Check sheet for the modelled part. Datum: model origin and axes. Units: mm. A direction names the side the tool comes from. Coordinates: 2 decimals unless noted, no trailing zeros. Write each loop counter-clockwise with the first axis right and the second up, starting at its lowest first coordinate (ties: lowest second). Pieces come first, ordered by that corner, then holes. Notation, with made-up numbers: (-32, 19.5) - (-22, 19.5) arc R15 ccw to (-22, 48.5) - close; hole circle Ø10 at (-28, 9.25). An arc over 180 degrees is marked (long way). Use one line per item in the form item = value. Start each with the question number.
1. Scan lines: line 1 along Y through (x, z) = (35.3, -15); line 2 along Y through (x, z) = (13, -10.5); line 3 along X through (y, z) = (7, -27). Record each from-to range of solid material in increasing order.
2. Cross-section at D-D on z = -19.75. Record the boundary of the cut face in (x, y), then the cut area to 3 significant figures.
3. Tool access check on faces 1 (the face through (22, 3, -15)), 2 (the face through (33.8, -12, -15)), 3 (the face through (3, 30.65, -15)). Record the directions out of +Z, -Z, +X, -X, +Y, -Y that give a thin tool (end or side, any length) a straight path to the whole face; none if there is none.
4. Draft check along Z on faces 4 (the face through (38.048, 2.287, -15.21)), 5 (the face through (15, 2, -30)), 6 (the face through (36.265, -5.159, -18.233)), 7 (the face through (2.47, 20.99, -13.26)). Enter one of: +Z half, -Z half, draft (parallel to the pull), parting line (faces both ways), or undercut.
5. Cross-section at A-A on y = 19.65. Record the boundary of the cut face in (x, z), then the cut area to 3 significant figures.
6. Go/stop test with flat-tipped pins: pin 1 Ø12.5 at (y, z) = (17, -18) entering from +X; pin 2 Ø14.5 at (x, z) = (19.5, -13.5) entering from +Y; pin 3 Ø1 at (x, z) = (14.5, -13.5) entering from -Y. Record where each tip stops, or that it passes through.
7. Cross-section at B-B on z = -15. Record the boundary of the cut face in (x, y), then the cut area to 3 significant figures.
8. Cross-section at C-C on y = -6.5. Record the boundary of the cut face in (x, z), then the cut area to 3 significant figures.
```python
from build123d import *

# Parameters (mm, degrees)
EXTRUDE_THIN1_DEPTH              = 30
F_7_0_7_DIAMETER_HOLE1_D         = 7
TAPPED_HOLE_FOR_8_32_HELICOIL1_D = 4.3942
SKETCH5_W                        = 43.8
SKETCH5_H                        = 32.238868154
EXTRUDE1_DEPTH                   = 31
FILLET1_R                        = 2.5


with BuildPart() as part:
    # Sketch1 → Extrude-Thin1 (new body)
    with BuildSketch(Plane.XY):
        Polygon((0, 30.65), (0, 0), (33.8, 0), (33.8, -20), (38.8, -20), (38.8, 5), (5, 5), (5, 30.65), align=None)
    extrude(amount=-EXTRUDE_THIN1_DEPTH)

    # Ø7.0 (7) Diameter Hole1 (through all)
    with Locations(Plane(origin=(38.8, -6.5, -15), x_dir=(0, 0, 1), z_dir=(1, 0, 0))):
        with Locations((0, 0)):
            Hole(F_7_0_7_DIAMETER_HOLE1_D / 2)

    # Tapped Hole for #8-32 Helicoil1 (through all)
    with Locations(Plane(origin=(5, 19.65, -15), x_dir=(0, 0, 1), z_dir=(1, 0, 0))):
        with Locations((0, 0)):
            Hole(TAPPED_HOLE_FOR_8_32_HELICOIL1_D / 2)

    # Sketch5 → Extrude1 (cut, through all)
    with BuildSketch(Plane.XY):
        with Locations((26.9, 19.119434077)):
            Rectangle(SKETCH5_W, SKETCH5_H)
    extrude(amount=-EXTRUDE1_DEPTH, mode=Mode.SUBTRACT)

    # Fillet1
    fillet1_edges = [part.edges().sort_by_distance(p)[0] for p in [
        (0, 0, -15),
        (38.8, 3, -15),
        (5, 3, -15),
    ]]
    fillet(fillet1_edges, radius=FILLET1_R)


solid = part.part
```
Final values:
q1.line_1 = -20 to -10, -3 to 3
q1.line_2 = 0 to 3
q1.line_3 = 0 to 5
q2.outline = (0, 2.5) arc R2.5 ccw to (2.5, 0) - (33.8, 0) - (33.8, -20) - (38.8, -20) - (38.8, 0.5) arc R2.5 ccw to (36.3, 3) - (7.5, 3) arc R2.5 cw to (5, 5.5) - (5, 30.65) - (0, 30.65) - close
q2.area = 353 mm²
q3.face_1 = +Z, -Z, +X, +Y
q3.face_2 = +Z, -Z, -X, -Y
q3.face_3 = +Z, -Z, +X, -X, +Y
q4.face_4 = draft
q4.face_5 = -Z half
q4.face_6 = undercut
q4.face_7 = undercut
q5.outline = (0, -30) - (5, -30) - (5, -17.2) - (0, -17.2) - close; (0, -12.8) - (5, -12.8) - (5, 0) - (0, 0) - close
q5.area = 128 mm²
q6.pin_1 = 5
q6.pin_2 = 3
q6.pin_3 = 0
q7.outline = (0, 2.5) arc R2.5 ccw to (2.5, 0) - (33.8, 0) - (33.8, -3) - (38.8, -3) - (38.8, 0.5) arc R2.5 ccw to (36.3, 3) - (7.5, 3) arc R2.5 cw to (5, 5.5) - (5, 17.45) - (0, 17.45) - close; (0, 21.85) - (5, 21.85) - (5, 30.65) - (0, 30.65) - close; (33.8, -20) - (38.8, -20) - (38.8, -10) - (33.8, -10) - close
q7.area = 296 mm²
q8.outline = (33.8, -30) - (38.8, -30) - (38.8, -18.5) - (33.8, -18.5) - close; (33.8, -11.5) - (38.8, -11.5) - (38.8, 0) - (33.8, 0) - close
q8.area = 115 mm²
